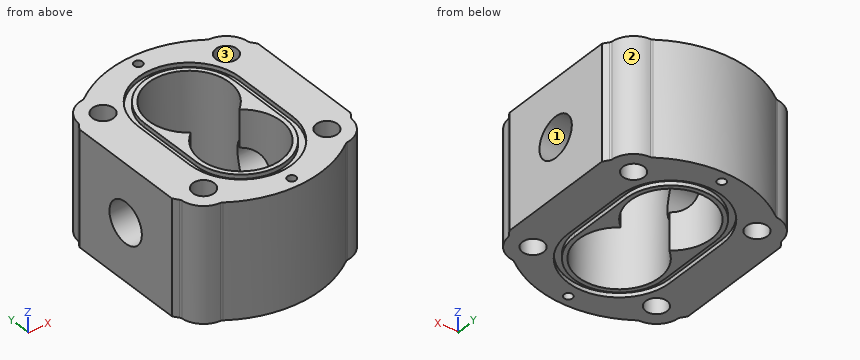
```python
from build123d import *

# Parameters (mm, degrees)
SKETCH2_R           = 5
BOSS_EXTRUDE1_DEPTH = 27
SKETCH3_R           = 9.5
CUT_EXTRUDE2_DEPTH  = 85
CUT_EXTRUDE3_DEPTH  = 2
SKETCH6_R           = 2
CUT_EXTRUDE4_DEPTH  = 3


with BuildPart() as part:
    # Sketch2 → Boss-Extrude1 (new body, symmetric)
    with BuildSketch(Plane.XY):
        with BuildLine():
            ThreePointArc((-39.949803133, 15.349672018), (-36.711412809, 22.144368202), (-29.86235622, 25.266145255))
            ThreePointArc((-29.86235622, 25.266145255), (-29.339100999, 25.379156062), (-28.864565634, 25.626913314))
            ThreePointArc((-28.864565634, 25.626913314), (0, 34.8), (28.864565634, 25.626913314))
            ThreePointArc((28.864565634, 25.626913314), (29.339100999, 25.379156062), (29.86235622, 25.266145255))
            ThreePointArc((29.86235622, 25.266145255), (36.711412809, 22.144368202), (39.949803133, 15.349672018))
            ThreePointArc((39.949803133, 15.349672018), (40.071741311, 14.828424908), (40.32757349, 14.358193726))
            ThreePointArc((40.32757349, 14.358193726), (41.181697345, 13.15608936), (42, 11.929319933))
            Line((42, 11.929319933), (42, -42.329319933))
            ThreePointArc((42, -42.329319933), (41.181697345, -43.55608936), (40.32757349, -44.758193726))
            ThreePointArc((40.32757349, -44.758193726), (40.071741311, -45.228424908), (39.949803133, -45.749672018))
            ThreePointArc((39.949803133, -45.749672018), (36.711412809, -52.544368202), (29.86235622, -55.666145255))
            ThreePointArc((29.86235622, -55.666145255), (29.339100999, -55.779156062), (28.864565634, -56.026913314))
            ThreePointArc((28.864565634, -56.026913314), (0, -65.2), (-28.864565634, -56.026913314))
            ThreePointArc((-28.864565634, -56.026913314), (-29.339100999, -55.779156062), (-29.86235622, -55.666145255))
            ThreePointArc((-29.86235622, -55.666145255), (-36.711412809, -52.544368202), (-39.949803133, -45.749672018))
            ThreePointArc((-39.949803133, -45.749672018), (-40.071741311, -45.228424908), (-40.32757349, -44.758193726))
            ThreePointArc((-40.32757349, -44.758193726), (-41.181697345, -43.55608936), (-42, -42.329319933))
            Line((-42, -42.329319933), (-42, 11.929319933))
            ThreePointArc((-42, 11.929319933), (-41.181697345, 13.15608936), (-40.32757349, 14.358193726))
            ThreePointArc((-40.32757349, 14.358193726), (-40.071741311, 14.828424908), (-39.949803133, 15.349672018))
        make_face()
        with Locations((-29, -44.7)):
            Circle(SKETCH2_R, mode=Mode.SUBTRACT)
        with Locations((-29, 14.3)):
            Circle(SKETCH2_R, mode=Mode.SUBTRACT)
        with Locations((29, -44.7)):
            Circle(SKETCH2_R, mode=Mode.SUBTRACT)
        with Locations((29, 14.3)):
            Circle(SKETCH2_R, mode=Mode.SUBTRACT)
        with BuildLine():
            ThreePointArc((-11.4, -15.2), (0, -49.4), (11.4, -15.2))
            ThreePointArc((11.4, -15.2), (0, 19), (-11.4, -15.2))
        make_face(mode=Mode.SUBTRACT)
    extrude(amount=BOSS_EXTRUDE1_DEPTH, both=True)

    # Sketch3 → Cut-Extrude2 (cut, through all)
    with BuildSketch(Plane(origin=(42, 0, 0), x_dir=(0, 0, -1), z_dir=(1, 0, 0))):
        with Locations((0, -15.2)):
            Circle(SKETCH3_R)
    extrude(amount=-CUT_EXTRUDE2_DEPTH, mode=Mode.SUBTRACT)

    # Sketch5 → Cut-Extrude3 (cut)
    with BuildSketch(Plane(origin=(0, 0, -27), x_dir=(-1, 0, 0), z_dir=(0, 0, -1))):
        with BuildLine():
            Line((-24, 0), (-24, -30.4))
            ThreePointArc((-24, -30.4), (0, -54.4), (24, -30.4))
            Line((24, -30.4), (24, 0))
            ThreePointArc((24, 0), (0, 24), (-24, 0))
        make_face()
        with BuildLine():
            Line((-21, 0), (-21, -30.4))
            ThreePointArc((-21, -30.4), (0, -51.4), (21, -30.4))
            Line((21, -30.4), (21, 0))
            ThreePointArc((21, 0), (0, 21), (-21, 0))
        make_face(mode=Mode.SUBTRACT)
    cut_extrude3 = extrude(amount=-CUT_EXTRUDE3_DEPTH, mode=Mode.SUBTRACT)

    # Sketch6 → Cut-Extrude4 (cut)
    with BuildSketch(Plane(origin=(0, 0, -27), x_dir=(-1, 0, 0), z_dir=(0, 0, -1))):
        with Locations((0, 29.8)):
            Circle(SKETCH6_R)
        with Locations((0, -60.2)):
            Circle(SKETCH6_R)
    cut_extrude4 = extrude(amount=-CUT_EXTRUDE4_DEPTH, mode=Mode.SUBTRACT)

    # Mirror1: Cut-Extrude3, Cut-Extrude4 across plane
    add(cut_extrude3.mirror(Plane.XY), mode=Mode.SUBTRACT)
    add(cut_extrude4.mirror(Plane.XY), mode=Mode.SUBTRACT)


solid = part.part
```
Input: part model. Units: mm. Frame: model coordinates. Face numbers are marked on the shaded views. Give positions to 0.01 mm unless a question says otherwise; leave off trailing zeros. Write each loop counter-clockwise with the first axis right and the second up, starting at its lowest first coordinate (ties: lowest second). Pieces come first, ordered by that corner, then holes. Notation, with made-up numbers: (15, 56) - (24, 56) arc R34 cw to (24, 91) - close; hole circle Ø4 at (-11, 86). An arc over 180 degrees is marked (long way). Write item = value, one per line. Start each with the question number.
1) Cut plane B-B (z = -22). Return loops of the section in (x, y), and give its area (3 significant figures).
2) Cut plane C-C (y = 8). Return loops of the section in (x, z), and give its area (3 significant figures).
3) Material intervals for L1, parallel to X at y = -46, z = 5; L2, parallel to Z at x = 31, y = -15; L3, parallel to X at y = 14, z = 12, sorted ascending. Write a range as [from, to].
4) Cut plane D-D (y = 29.8). Return loops of the section in (x, z), and give its area (3 significant figures).
5) Cut plane A-A (z = 0). Give the number of separate pieces and of enclosed holes in the cut face, and give its area (3 significant figures).
6) Pin query (flat end, axial travel): pin 1 (24.5 mm diameter, centred on y = -15.2, z = 0, fed in from +X); pin 2 (1 mm diameter, centred on x = -15, z = -8.5, fed in from +Y); pin 3 (8 mm diameter, centred on x = 17.5, z = -13, fed in from +Y); pin 4 (10 mm diameter, centred on x = 30.5, z = 5.5, fed in from -Y). Return the tip coordinate at first contact, or that it passes through.
7) Draft query along X for the marked faces 1, 2 and 3. Return one class per face: pulls with the +X half, pulls with the -X half, needs draft (parallel to the pull), parting line crosses it, or undercut.
Answers follow:
q1.outline = (-42, -42.33) arc R50 ccw to (-40.33, -44.76) arc R2 cw to (-39.95, -45.75) arc R11 ccw to (-29.86, -55.67) arc R2 cw to (-28.86, -56.03) arc R50 ccw to (28.86, -56.03) arc R2 cw to (29.86, -55.67) arc R11 ccw to (39.95, -45.75) arc R2 cw to (40.33, -44.76) arc R50 ccw to (42, -42.33) - (42, 11.93) arc R50 ccw to (40.33, 14.36) arc R2 cw to (39.95, 15.35) arc R11 ccw to (29.86, 25.27) arc R2 cw to (28.86, 25.63) arc R50 ccw to (-28.86, 25.63) arc R2 cw to (-29.86, 25.27) arc R11 ccw to (-39.95, 15.35) arc R2 cw to (-40.33, 14.36) arc R50 ccw to (-42, 11.93) - close; hole circle Ø10 at (-29, -44.7); hole circle Ø10 at (-29, 14.3); hole (-11.4, -15.2) arc R19 ccw (long way) to (11.4, -15.2) arc R19 ccw (long way) to start; hole circle Ø10 at (29, -44.7); hole circle Ø10 at (29, 14.3)
q1.area = 4,900 mm^2
q2.outline = (-42, -27) - (-22.63, -27) - (-22.63, -25) - (-19.42, -25) - (-19.42, -27) - (-17.23, -27) - (-17.23, 27) - (-19.42, 27) - (-19.42, 25) - (-22.63, 25) - (-22.63, 27) - (-42, 27) - close; (17.23, -27) - (19.42, -27) - (19.42, -25) - (22.63, -25) - (22.63, -27) - (42, -27) - (42, 27) - (22.63, 27) - (22.63, 25) - (19.42, 25) - (19.42, 27) - (17.23, 27) - close
q2.area = 2,650 mm^2
q3.L1 = [-39.92, -33.83], [-24.17, -10.85], [10.85, 24.17], [33.83, 39.92]
q3.L2 = [-27, -9.5], [9.5, 27]
q3.L3 = [-40.59, -33.99], [-24.01, -12.85], [12.85, 24.01], [33.99, 40.59]
q4.outline = (-21.79, -27) - (-2, -27) - (-2, -24) - (2, -24) - (2, -27) - (21.79, -27) - (21.79, 27) - (2, 27) - (2, 24) - (-2, 24) - (-2, 27) - (-21.79, 27) - close
q4.area = 2,330 mm^2
q5.separate_pieces = 2
q5.enclosed_holes = 4
q5.area = 3,890 mm^2
q6.pin_1 = 42
q6.pin_2 = 32.65
q6.pin_3 = 32.94
q6.pin_4 = -58.21
q7.face_1 = needs draft
q7.face_2 = pulls with the +X half
q7.face_3 = undercut
